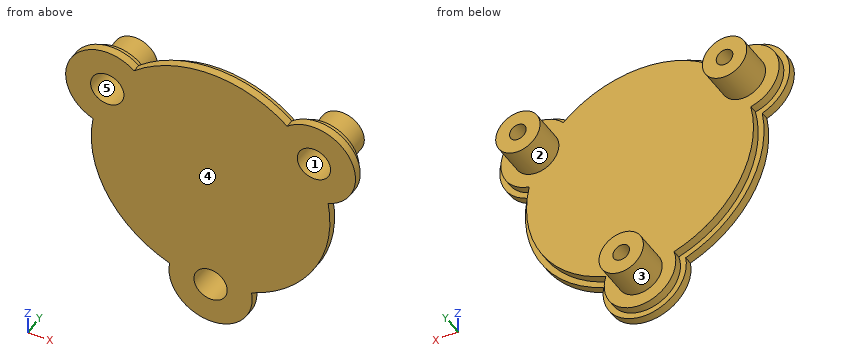
from build123d import *

# Parameters (mm, degrees)
SKETCH1_R           = 6
BOSS_EXTRUDE1_DEPTH = 3
SKETCH1_3_R         = 8
SKETCH1_3_R_2       = 6
BOSS_EXTRUDE2_DEPTH = 18
SKETCH2_R           = 8
BOSS_EXTRUDE3_DEPTH = 3
SKETCH3_R           = 6
SKETCH3_R_2         = 3
BOSS_EXTRUDE4_DEPTH = 6


with BuildPart() as part:
    # Sketch1 → Boss-Extrude1 (new body)
    with BuildSketch(Plane(origin=(0, 0, 0), x_dir=(1, 0, 0), z_dir=(0, 1, 0))):
        with BuildLine():
            ThreePointArc((42.358365189, -7.400601228), (37.239092363, 21.5), (14.770073928, 40.38372093))
            ThreePointArc((14.770073928, 40.38372093), (0, 58), (-14.770073928, 40.38372093))
            ThreePointArc((-14.770073928, 40.38372093), (-37.239092363, 21.5), (-42.358365189, -7.400601228))
            ThreePointArc((-42.358365189, -7.400601228), (-50.229473419, -29), (-27.588291261, -32.983119702))
            ThreePointArc((-27.588291261, -32.983119702), (0, -43), (27.588291261, -32.983119702))
            ThreePointArc((27.588291261, -32.983119702), (50.22947342, -29), (42.358365189, -7.400601228))
        make_face()
        with Locations((-37.239092363, -21.5)):
            Circle(SKETCH1_R, mode=Mode.SUBTRACT)
        with Locations((0, 43)):
            Circle(SKETCH1_R, mode=Mode.SUBTRACT)
        with Locations((37.239092363, -21.5)):
            Circle(SKETCH1_R, mode=Mode.SUBTRACT)
    extrude(amount=BOSS_EXTRUDE1_DEPTH)

    # Sketch1_3 → Boss-Extrude2 (add)
    with BuildSketch(Plane(origin=(0, 0, 0), x_dir=(1, 0, 0), z_dir=(0, 1, 0))):
        with Locations((0, 43)):
            Circle(SKETCH1_3_R)
        with Locations((0, 43)):
            Circle(SKETCH1_3_R_2, mode=Mode.SUBTRACT)
        with Locations((37.239092363, -21.5)):
            Circle(SKETCH1_3_R)
        with Locations((37.239092363, -21.5)):
            Circle(SKETCH1_3_R_2, mode=Mode.SUBTRACT)
        with Locations((-37.239092363, -21.5)):
            Circle(SKETCH1_3_R)
        with Locations((-37.239092363, -21.5)):
            Circle(SKETCH1_3_R_2, mode=Mode.SUBTRACT)
    extrude(amount=BOSS_EXTRUDE2_DEPTH)

    # Sketch2 → Boss-Extrude3 (add)
    with BuildSketch(Plane(origin=(0, 3, 0), x_dir=(1, 0, 0), z_dir=(0, 1, 0))):
        with BuildLine():
            ThreePointArc((39.923825333, -8.882464231), (35.420439015, 20.45), (12.269472994, 39.01627907))
            ThreePointArc((12.269472994, 39.01627907), (0, 55.9), (-12.269472994, 39.01627907))
            ThreePointArc((-12.269472994, 39.01627907), (-35.420439015, 20.45), (-39.923825333, -8.882464231))
            ThreePointArc((-39.923825333, -8.882464231), (-48.410820072, -27.95), (-27.654352339, -30.133814839))
            ThreePointArc((-27.654352339, -30.133814839), (0, -40.9), (27.654352339, -30.133814839))
            ThreePointArc((27.654352339, -30.133814839), (48.410820072, -27.95), (39.923825333, -8.882464231))
        make_face()
        with Locations((37.239092363, -21.5)):
            Circle(SKETCH2_R, mode=Mode.SUBTRACT)
        with Locations((0, 43)):
            Circle(SKETCH2_R, mode=Mode.SUBTRACT)
        with Locations((-37.239092363, -21.5)):
            Circle(SKETCH2_R, mode=Mode.SUBTRACT)
    extrude(amount=BOSS_EXTRUDE3_DEPTH)

    # Sketch3 → Boss-Extrude4 (add)
    with BuildSketch(Plane(origin=(0, 18, 0), x_dir=(1, 0, 0), z_dir=(0, 1, 0))):
        with Locations((-37.239092363, -21.5)):
            Circle(SKETCH3_R)
        with Locations((-37.239092363, -21.5)):
            Circle(SKETCH3_R_2, mode=Mode.SUBTRACT)
        with Locations((0, 43)):
            Circle(SKETCH3_R)
        with Locations((0, 43)):
            Circle(SKETCH3_R_2, mode=Mode.SUBTRACT)
        with Locations((37.239092363, -21.5)):
            Circle(SKETCH3_R)
        with Locations((37.239092363, -21.5)):
            Circle(SKETCH3_R_2, mode=Mode.SUBTRACT)
    extrude(amount=-BOSS_EXTRUDE4_DEPTH)


solid = part.part
Could you check a few things on this model? Use its own coordinates, in mm. Face numbers are marked on the shaded views. A direction names the side the tool comes from. Give positions to 0.01 mm unless a question says otherwise; leave off trailing zeros. Order: outer loops, then holes, each group sorted by start corner. A loop starts at its lowest first (then second) coordinate and runs counter-clockwise, first axis right, second up.
1. Suppose I cut it at B-B (x = 0). Write out the boundary of the cut face in (y, z), plus the area to 3 significant figures.
Answers below:
outline: (0, -58) - (3, -58) - (3, -55.9) - (6, -55.9) - (6, -51) - (18, -51) - (18, -46) - (12, -46) - (12, -49) - (0, -49) - close; (0, -37) - (12, -37) - (12, -40) - (18, -40) - (18, -35) - (6, -35) - (6, 40.9) - (3, 40.9) - (3, 43) - (0, 43) - close
area: 605 mm2
2. For pin 1 (11 mm diameter, centred on x = -37.24, z = 21.5, fed in from -Y); pin 2 (8 mm diameter, centred on x = -9, y = 9, fed in from -Z); pin 3 (10 mm diameter, centred on y = 6.5, z = -2.5, fed in from +X), each with a flat end and sliding along its axis, tell me the tip position at first contact or that it passes through.
Answers below:
pin 1: stops at y = 12
pin 2: stops at z = -54.23
pin 3: stops at x = 43
3. I need wall thicknesses on L1, parallel to X at y = 3.25, z = 21.5; L2, parallel to X at y = 14.85, z = -43; L3, parallel to X at y = 5, z = -43. Which ranges of each line are inside material? Lowest first, please.
Answers below:
L1: x = -50.14 to -43.24, -31.24 to 31.24, 43.24 to 50.14
L2: x = -8 to -3, 3 to 8
L3: x = -12.9 to -6, 6 to 12.9
4. Thinking about a two-plate mould opening in X: for the marked faces 3, 4 and 5, which applies, +X half, -X half, draft (parallel to the pull), parting line (faces both ways), or undercut?
Answers below:
face 3: parting line
face 4: draft
face 5: undercut
5. Suppose I cut it at C-C (y = 13.75). Write out the boundary of the cut face in (x, z).
Answers below:
outline: circle Ø16 at (-37.24, 21.5); circle Ø16 at (0, -43); circle Ø16 at (37.24, 21.5); hole circle Ø6 at (-37.24, 21.5); hole circle Ø6 at (0, -43); hole circle Ø6 at (37.24, 21.5)
6. Suppose I cut it at D-D (z = -43). Write out the boundary of the cut face in (x, y), plus the area to 3 significant figures.
Answers below:
outline: (-15, 0) - (-6, 0) - (-6, 12) - (-3, 12) - (-3, 18) - (-8, 18) - (-8, 6) - (-12.9, 6) - (-12.9, 3) - (-15, 3) - close; (3, 12) - (6, 12) - (6, 0) - (15, 0) - (15, 3) - (12.9, 3) - (12.9, 6) - (8, 6) - (8, 18) - (3, 18) - close
area: 179 mm2
7. Suppose I cut it at A-A (z = 21.5). State how many separate pieces and enclosed holes the cut face has, plus the area to 3 significant figures.
Answers below:
separate pieces: 3
enclosed holes: 0
area: 638 mm2
8. Which directions (+Z, -Z, +X, -X, +Y, -Y) give clear straight access to the entire face, cutting with the end or side of a thin tool? Please do the marked faces 1 and 2.
Answers below:
face 1: -Y
face 2: +Y
